For this review, take the finished solid that the model builds, in its own axes (mm). Give positions to 0.01 mm unless a question says otherwise; leave off trailing zeros. Loops run counter-clockwise (first coordinate to the right, second up) from the corner with the lowest first, then second, coordinate; pieces in that order, holes last. Notation, with made-up numbers: (59.25, 66.5) - (108.25, 66.5) arc R22 ccw to (108.25, 81.5) - close; hole circle Ø4 at (10, 40). An arc over 180 degrees is marked (long way). Use CSV: the item, a comma, the result in double quotes. Start each with the question number.
1. Take a section at A-A on x = -14.5. Give the boundary of the cut face in (y, z).
2. Take a section at C-C on x = 2. Give the boundary of the cut face in (y, z).
3. For pin 1 (6.5 mm diameter, centred on x = -2.53, y = -4, fed in from +Z); pin 2 (4 mm diameter, centred on x = 15.36, y = 11.01, fed in from +Z), all flat-tipped, find the tip position at first contact; note any pin that passes through.
4. Wall thickness on line 1 (Y direction, x = 0, z = 11.25); line 2 (Y direction, x = -3.5, z = 3); line 3 (Y direction, x = -1, z = 18.75): over which ranges is each line inside the solid? List them lowest first.
5. Mouldability with a two-part tool opening along Y and no side actions: class faces 1 (the flat face through (0, 0, 0)), 2 (the flat face through (0, 25, 12)), 3 (the cylindrical face through (9.126, -3.494, 12.325)) as pulls with the +Y half, pulls with the -Y half, needs draft (parallel to the pull), parting line crosses it, or undercut.
6. Take a section at B-B on z = 8.75. Give the boundary of the cut face in (x, y), plus the area to 3 significant figures.
```python
from build123d import *

# Parameters (mm, degrees)
F0_W     = 50
F0_H     = 50
F1_DEPTH = 25
F3_D     = 10.3
F4_D     = 8.5
F5_D     = 6.8
F6_D     = 5
F7_D     = 4.2
F8_D     = 3.3
F9_D     = 2.5


with BuildPart() as f1:
    # F0 (on Top) → F1 (new body)
    with BuildSketch(Plane.XY):
        Rectangle(F0_W, F0_H)
    extrude(amount=F1_DEPTH)

    # F3 (through all)
    with Locations(Plane.XY.offset(25)):
        with Locations((-13.114403002, 10.6317354366)):
            Hole(F3_D / 2)

    # F4 (through all)
    with Locations(Plane.XY.offset(25)):
        with Locations((0, 11.0131110996)):
            Hole(F4_D / 2)

    # F5 (through all)
    with Locations(Plane.XY.offset(25)):
        with Locations((15.3620382771, 11.0131110996)):
            Hole(F5_D / 2)

    # F6 (through all)
    with Locations(Plane.XY.offset(25)):
        with Locations((-14.8614421487, -5.0685340539)):
            Hole(F6_D / 2)

    # F7 (through all)
    with Locations(Plane.XY.offset(25)):
        with Locations((-2.5342670269, -4.0047676302)):
            Hole(F7_D / 2)

    # F8 (through all)
    with Locations(Plane.XY.offset(25)):
        with Locations((7.4776518159, -3.5667461343)):
            Hole(F8_D / 2)

    # F9 (through all)
    with Locations(Plane.XY.offset(25)):
        with Locations((15.8626344055, -2.5029797107)):
            Hole(F9_D / 2)


solid = f1.part
```
Check result:
1,outline,"(-25, 0) - (-7.54, 0) - (-7.54, 25) - (-25, 25) - close; (-2.59, 0) - (5.67, 0) - (5.67, 25) - (-2.59, 25) - close; (15.59, 0) - (25, 0) - (25, 25) - (15.59, 25) - close"
2,outline,"(-25, 0) - (7.26, 0) - (7.26, 25) - (-25, 25) - close; (14.76, 0) - (25, 0) - (25, 25) - (14.76, 25) - close"
3,pin 1,"stops at z = 25"
3,pin 2,"passes through"
4,line 1,"y = -25 to 6.76, 15.26 to 25"
4,line 2,"y = -25 to -5.87, -2.14 to 8.6, 13.42 to 25"
4,line 3,"y = -25 to -5.44, -2.57 to 6.88, 15.14 to 25"
5,face 1,"needs draft"
5,face 2,"pulls with the +Y half"
5,face 3,"undercut"
6,outline,"(-25, -25) - (25, -25) - (25, 25) - (-25, 25) - close; hole circle Ø10.3 at (-13.11, 10.63); hole circle Ø5 at (-14.86, -5.07); hole circle Ø4.2 at (-2.53, -4); hole circle Ø8.5 at (0, 11.01); hole circle Ø3.3 at (7.48, -3.57); hole circle Ø6.8 at (15.36, 11.01); hole circle Ø2.5 at (15.86, -2.5)"
6,area,"2,280 mm²"
